CAD build for the part. Positions are in the model's coordinates, mm. A direction names the side the tool comes from. Give positions to 0.01 mm unless a question says otherwise; leave off trailing zeros. Loops run counter-clockwise (first coordinate to the right, second up) from the corner with the lowest first, then second, coordinate; pieces in that order, holes last. Notation, with made-up numbers: (77.5, 12.25) - (87.5, 12.25) arc R20 ccw to (87.5, 51.25) - close; hole circle Ø4 at (-37.5, -11). An arc over 180 degrees is marked (long way). Return JSON: item names as keys, results as strings.
from build123d import *

# Parameters (mm, degrees)
SKETCH1_R                = 5.715
BOSS_EXTRUDE1_DEPTH      = 25.4
BOSS_EXTRUDE3_DEPTH      = 6.35
BOSS_EXTRUDE4_DEPTH      = 11.430000000000001
BOSS_EXTRUDE4_DEPTH_BACK = 19.05
CUT_EXTRUDE1_START       = -19.05
SKETCH5_R                = 28.575000000000006
CUT_EXTRUDE1_DEPTH       = 19.05


with BuildPart() as part:
    # Sketch1 → Boss-Extrude1 (new body)
    with BuildSketch(Plane(origin=(0, 0, 0), x_dir=(1, 0, 0), z_dir=(0, 1, 0))):
        with Locations(Location((0, 0, 0), (0, 0, 270))):
            Circle(SKETCH1_R)
        with BuildLine():
            Line((3.801523904962324, -2.54), (-3.801523904962324, -2.54))
            ThreePointArc((-3.8015239049623246, -2.5400000000000005), (-1.33e-15, 4.572000000000001), (3.801523904962326, -2.5399999999999983))
        make_face(mode=Mode.SUBTRACT)
    extrude(amount=BOSS_EXTRUDE1_DEPTH)

    # Sketch2 → Boss-Extrude3 (add)
    with BuildSketch(Plane(origin=(0, 25.4, 0), x_dir=(1, 0, 0), z_dir=(0, 1, 0))):
        with BuildLine():
            Line((3.801523904962324, -2.54), (-3.801523904962324, -2.54))
            ThreePointArc((-3.8015239049623246, -2.5400000000000005), (-4.572, 5.607e-14), (-3.801523904962262, 2.540000000000094))
            Line((-3.801523904962324, 2.540000000000111), (-3.801523904962324, 4.267275594568456))
            ThreePointArc((-3.801523904962365, 4.26727559456847), (-2.338323746098912, -5.214735569367823), (5.715, -1.4e-15))
            ThreePointArc((5.715, 0), (5.214735569367823, 2.338323746098912), (3.801523904962363, 4.267275594568472))
            Line((3.801523904962324, 4.267275594568458), (3.801523904962324, 2.5400000000001137))
            ThreePointArc((3.801523904962324, 2.540000000000001), (4.572000000000001, 1.44e-15), (3.801523904962326, -2.5399999999999983))
        make_face()
        with BuildLine():
            Line((-3.801523904962324, 2.540000000000111), (-3.801523904962324, -2.54))
            Line((-3.801523904962324, -2.54), (3.801523904962324, -2.54))
            Line((3.801523904962324, -2.54), (3.801523904962324, 2.5400000000001137))
            ThreePointArc((3.801523904962324, 2.540000000000001), (5.507e-14, 4.572000000000001), (-3.801523904962262, 2.540000000000094))
        make_face()
        with BuildLine():
            Line((-3.801523904962324, 32.590628837493085), (-3.801523904962324, 4.267275594568456))
            ThreePointArc((-3.801523904962365, 4.26727559456847), (-2.19e-15, 5.715), (3.801523904962363, 4.267275594568472))
            Line((3.801523904962324, 4.267275594568458), (3.801523904962324, 32.590628837493085))
            Line((3.801523904962324, 32.590628837493085), (-3.801523904962324, 32.590628837493085))
        make_face()
        with BuildLine():
            Line((-3.801523904962324, 4.267275594568456), (-3.801523904962324, 2.540000000000111))
            ThreePointArc((-3.801523904962262, 2.540000000000094), (5.507e-14, 4.572000000000001), (3.801523904962324, 2.540000000000001))
            Line((3.801523904962324, 2.5400000000001137), (3.801523904962324, 4.267275594568458))
            ThreePointArc((3.801523904962363, 4.267275594568472), (-2.19e-15, 5.715), (-3.801523904962365, 4.26727559456847))
        make_face()
        with BuildLine():
            ThreePointArc((-3.801523904962262, 2.540000000000094), (-4.572, 5.607e-14), (-3.8015239049623246, -2.5400000000000005))
            Line((-3.801523904962324, -2.54), (-3.801523904962324, 2.540000000000111))
        make_face()
        with BuildLine():
            Line((3.801523904962324, 2.5400000000001137), (3.801523904962324, -2.54))
            ThreePointArc((3.801523904962326, -2.5399999999999983), (4.572000000000001, 1.44e-15), (3.801523904962324, 2.540000000000001))
        make_face()
    extrude(amount=BOSS_EXTRUDE3_DEPTH)

    # Sketch4 → Boss-Extrude4 (add, two sides: drawn at the far end of the back side and taken through both)
    with BuildSketch(Plane.ZY.offset(3.801523904962324).offset(-BOSS_EXTRUDE4_DEPTH_BACK)):
        with BuildLine():
            Line((-64.34062883749309, 12.723017723708097), (-61.16562883749309, 12.723017723708097))
            ThreePointArc((-61.16562883749309, 12.7230177237081), (-42.772401198467776, 39.4224959318921), (-11.27151604034228, 31.75000000000092))
            Line((-11.271516040342593, 31.75), (-7.173381829650392, 31.75))
            ThreePointArc((-7.173381829650484, 31.74999999999974), (-42.61721618067714, 42.8482570795954), (-64.34062883749309, 12.7230177237081))
        make_face()
        with BuildLine():
            Line((-7.173381829650392, 31.75), (-11.271516040342593, 31.75))
            ThreePointArc((-11.27151604034228, 31.75000000000092), (-8.912699493419062, 28.719463797040717), (-6.981553388219599, 25.39999999999997))
            Line((-6.9815533882195915, 25.4), (-4.267275594568506, 25.4))
            Line((-4.267275594568505, 25.4), (-4.267275594568505, 27.07049698232741))
            ThreePointArc((-4.267275594568467, 27.07049698232742), (-5.618653271152166, 29.473391870237137), (-7.173381829650484, 31.74999999999974))
        make_face()
    extrude(amount=BOSS_EXTRUDE4_DEPTH + BOSS_EXTRUDE4_DEPTH_BACK)

    # Sketch5 → Cut-Extrude1 (cut)
    with BuildSketch(Plane.ZY.offset(3.801523904962324).offset(CUT_EXTRUDE1_START)):
        with Locations((-32.590628837493085, 12.723017723708097)):
            Circle(SKETCH5_R)
    extrude(amount=CUT_EXTRUDE1_DEPTH, mode=Mode.SUBTRACT)


solid = part.part
1. Pull direction Z, two halves, no side cores. Call faces 6 (the face through (0, 0, 3)), 7 (the face through (0.22, 40.42, -39.62)): +Z half, -Z half, draft (parallel to the pull), parting line (faces both ways), or undercut.
Values follow:
{"face 6": "draft", "face 7": "undercut"}
2. Cut at B-B, the plane z = 0. Write the cut outline in (x, y) (3 decimals), plus the area to 3 significant figures.
Values follow:
{"outline": "(-5.715, 0) - (-4.572, 0) - (-4.572, 25.4) - (4.572, 25.4) - (4.572, 0) - (5.715, 0) - (5.715, 31.75) - (-5.715, 31.75) - close", "area": "131 mm²"}
3. Which spindle directions (+Z, -Z, +X, -X, +Y, -Y) get a long thin tool onto all of the face, cutting with end or side? Do faces 1 (the face through (0, 13, 2.54)), 2 (the face through (3.802, 30, -5)), 3 (the face through (-3.802, 30, -5)), 4 (the face through (-9, 26, -4.267)), 5 (the face through (0, 12.723, -63)). Say none if no direction does.
Values follow:
{"face 1": "-Y", "face 2": "+X, +Y", "face 3": "-X, +Y", "face 4": "-X, +Y, -Y", "face 5": "-Z, +X, -X, -Y"}
4. Cut at A-A, the plane x = 0. Write the cut outline in (y, z) (3 decimals).
Values follow:
{"outline": "(0, -5.715) - (3.016, -5.715) arc R28.575 cw to (7.112, -4.572) - (0, -4.572) - close; (0, 2.54) - (25.4, 2.54) - (25.4, -4.572) - (18.334, -4.572) arc R28.575 cw to (22.43, -5.715) - (25.4, -5.715) - (25.4, -6.982) arc R28.575 cw to (12.723, -61.166) - (12.723, -64.341) arc R31.75 ccw to (31.75, -7.173) - (31.75, 5.715) - (0, 5.715) - close"}
5. Cut at C-C, the plane y = 36.5. Write the cut outline in (x, z), plus the area to 3 significant figures.
Values follow:
{"outline": "(-15.23, -53.63) - (15.25, -53.63) - (15.25, -48.44) - (-15.23, -48.44) - close; (-15.23, -16.74) - (15.25, -16.74) - (15.25, -11.55) - (-15.23, -11.55) - close", "area": "317 mm²"}
6. Cut at D-D, the plane y = 10. Write the cut outline in (x, z) (3 decimals).
Values follow:
{"outline": "(-3.802, -4.267) - (-3.802, -4.146) - (-1.928, -4.146) arc R4.572 cw to (-3.802, 2.54) - (3.802, 2.54) arc R4.572 cw to (1.928, -4.146) - (3.934, -4.146) arc R5.715 ccw (long way) to start"}
7. Drop flat-ended pins along their axis: P1, Ø6, axis at x = 5, y = 10, coming from the +Z side; P2, Ø3.5, axis at x = 1.5, z = -2, coming from the -Y side; P3, Ø1, axis at x = -8, z = -30.5, coming from the +Y side. Give the stop position or say it passes through.
Values follow:
{"P1": "stops at z = 5.35", "P2": "stops at y = 25.4", "P3": "stops at y = 44.43"}
8. Drill centre lines: probe 1 along X at (y, z) = (19.5, 0) (3 decimals); probe 2 along Z at (x, y) = (0, 5.75) (3 decimals); probe 3 along Z at (x, y) = (0, 13.75) (3 decimals). Where is each one in solid material? Low to high.
Values follow:
{"probe 1": "x = -5.715 to -4.572, 4.572 to 5.715", "probe 2": "z = -4.879 to -4.572, 2.54 to 5.715", "probe 3": "z = -64.324 to -61.147, 2.54 to 5.715"}
